Geometry check sheet. Reference: the model listing, model coordinates, mm. Face numbers are marked on the shaded views. Coordinates: 2 decimals unless noted, no trailing zeros. Write each loop counter-clockwise with the first axis right and the second up, starting at its lowest first coordinate (ties: lowest second). Pieces come first, ordered by that corner, then holes. Notation, with made-up numbers: (-7, -1) -> (32, -1) arc R27 ccw to (32, 31) -> close; hole circle Ø3 at (74, 15.25). An arc over 180 degrees is marked (long way). Answer as CSV lines item,"result".
```python
from build123d import *

# Parameters (mm, degrees)
F0_W     = 127
F0_H     = 127
F1_DEPTH = 127
F2_R     = 12.7
F3_SIZE  = 12.7
F5_R     = 25.4
F6_DEPTH = 127.001


with BuildPart() as f1:
    # F0 (on Front) → F1 (new body)
    with BuildSketch(Plane.XZ):
        with Locations((0.102586, 63.5)):
            Rectangle(F0_W, F0_H)
    extrude(amount=F1_DEPTH)

    # F2
    f2_edges = [f1.edges().sort_by_distance(p)[0] for p in [
        (-63.397414, -63.5, 127),
    ]]
    fillet(f2_edges, radius=F2_R)

    # F3
    f3_edges = [f1.edges().sort_by_distance(p)[0] for p in [
        (63.602586, -63.5, 127),
    ]]
    chamfer(f3_edges, length=F3_SIZE)

    # F5 (on face) → F6 (cut, through all)
    with BuildSketch(Plane.XZ.offset(127)):
        with Locations((0, 56.165393)):
            Circle(F5_R)
    extrude(amount=-F6_DEPTH, mode=Mode.SUBTRACT)


solid = f1.part
```
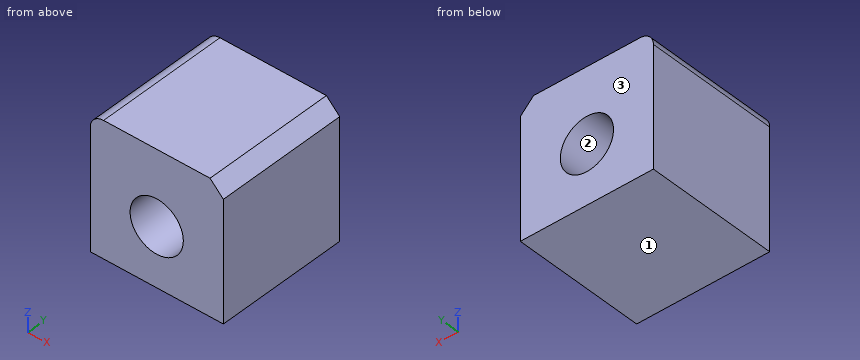
Item 1: Thickness scan on probe 1 along Z at (x, y) = (0, -46); probe 2 along X at (y, z) = (-28, 74); probe 3 along X at (y, z) = (-74, 63.5). Record the ranges inside material, lowest first.
Responses:
probe 1,"z = 0 to 30.77, 81.57 to 127"
probe 2,"x = -63.4 to -18.09, 18.09 to 63.6"
probe 3,"x = -63.4 to -24.32, 24.32 to 63.6"
Item 2: Cross-section at A-A, the plane x = 0. Record the cut outline in (y, z).
Responses:
outline,"(-127, 0) -> (0, 0) -> (0, 30.77) -> (-127, 30.77) -> close; (-127, 81.57) -> (0, 81.57) -> (0, 127) -> (-127, 127) -> close"
Item 3: Release check for a two-part mould opening along Z. For the marked faces 1, 2 and 3 record: +Z half, -Z half, draft (parallel to the pull), parting line (faces both ways), or undercut.
Responses:
face 1,"-Z half"
face 2,"undercut"
face 3,"draft"
Item 4: Cross-section at C-C, the plane y = -25.5. Record the cut outline in (x, z), plus the area to 3 significant figures.
Responses:
outline,"(-63.4, 0) -> (63.6, 0) -> (63.6, 114.3) -> (50.9, 127) -> (-50.7, 127) arc R12.7 ccw to (-63.4, 114.3) -> close; hole circle Ø50.8 at (0, 56.17)"
area,"14,000 mm2"
Item 5: Cross-section at B-B, the plane z = 45. Record the cut outline in (x, y), plus the area to 3 significant figures.
Responses:
outline,"(-63.4, -127) -> (-22.81, -127) -> (-22.81, 0) -> (-63.4, 0) -> close; (22.81, -127) -> (63.6, -127) -> (63.6, 0) -> (22.81, 0) -> close"
area,"10,300 mm2"
